Source: CAD feature listing. Evaluate the final solid. Frame: model axes, mm. A direction names the side the tool comes from. Give positions to 0.01 mm unless a question says otherwise; leave off trailing zeros. Loops run counter-clockwise (first coordinate to the right, second up) from the corner with the lowest first, then second, coordinate; pieces in that order, holes last. Notation, with made-up numbers: M 10,43.5 L 31,43.5 A30 ccw 31,77.5 Z; hole C 68,65 d9. An arc over 180 degrees is marked long. Answer in a Markdown table with one row per item.
```python
from build123d import *

# Parameters (mm, degrees)
SKETCH1_W           = 104
SKETCH1_H           = 6
BOSS_EXTRUDE1_DEPTH = 5
SKETCH2_W           = 104
SKETCH2_H           = 3
BOSS_EXTRUDE2_DEPTH = 92
SKETCH3_W           = 5
SKETCH3_H           = 6
BOSS_EXTRUDE3_DEPTH = 3
SKETCH4_W           = 5
SKETCH4_H           = 6
BOSS_EXTRUDE4_DEPTH = 3


with BuildPart() as part:
    # Sketch1 → Boss-Extrude1 (new body)
    with BuildSketch(Plane.XY):
        Rectangle(SKETCH1_W, SKETCH1_H)
    extrude(amount=-BOSS_EXTRUDE1_DEPTH)

    # Sketch2 → Boss-Extrude2 (add)
    with BuildSketch(Plane(origin=(0, 0, -5), x_dir=(-1, 0, 0), z_dir=(0, 0, -1))):
        with Locations((0, -1.5)):
            Rectangle(SKETCH2_W, SKETCH2_H)
    extrude(amount=BOSS_EXTRUDE2_DEPTH)

    # Sketch3 → Boss-Extrude3 (add)
    with BuildSketch(Plane(origin=(52, 0, 0), x_dir=(0, 0, -1), z_dir=(1, 0, 0))):
        with Locations((2.5, 0)):
            Rectangle(SKETCH3_W, SKETCH3_H)
    extrude(amount=BOSS_EXTRUDE3_DEPTH)

    # Sketch4 → Boss-Extrude4 (add)
    with BuildSketch(Plane.ZY.offset(52)):
        with Locations((-2.5, 0)):
            Rectangle(SKETCH4_W, SKETCH4_H)
    extrude(amount=BOSS_EXTRUDE4_DEPTH)


solid = part.part
```
1) Pin query (flat end, axial travel): pin 1 Ø3.5 at (y, z) = (-2, -58.5) entering from +X; pin 2 Ø4 at (x, z) = (40, -62.5) entering from +Y; pin 3 Ø2.5 at (y, z) = (-1.5, -69.5) entering from -X; pin 4 Ø2 at (x, y) = (20, 1.5) entering from +Z. Return the tip coordinate at first contact, or that it passes through.
Reply:
| item | result |
|---|---|
| pin 1 | stops at x = 52 |
| pin 2 | stops at y = 0 |
| pin 3 | stops at x = -52 |
| pin 4 | stops at z = 0 |
2) Section B-B, the plane x = 41. Return loops of the section in (y, z).
Reply:
| item | result |
|---|---|
| outline | M -3,-97 L 0,-97 L 0,-5 L 3,-5 L 3,0 L -3,0 Z |
3) Material intervals for L1, parallel to Y at x = -32, z = -50.5; L2, parallel to X at y = -0.9, z = -86; L3, parallel to Z at x = -48.5, y = 1.8, sorted ascending.
Reply:
| item | result |
|---|---|
| L1 | y = -3 to 0 |
| L2 | x = -52 to 52 |
| L3 | z = -5 to 0 |
4) Section A-A, the plane y = -1.5. Return loops of the section in (x, z), then the cut area to 3 significant figures.
Reply:
| item | result |
|---|---|
| outline | M -55,-5 L -52,-5 L -52,-97 L 52,-97 L 52,-5 L 55,-5 L 55,0 L -55,0 Z |
| area | 10,100 mm² |
5) Set-up query: faces 1 (the flat face through (1, 0, -50)), 2 (the flat face through (1, -3, -49)), 3 (the flat face through (-52, -2, -50)), 4 (the flat face through (52, -2, -50)), 5 (the flat face through (55, 0, -2)). Return all of +Z, -Z, +X, -X, +Y, -Y with unobstructed straight access to the full face (end or side cutting, diameter ignored); none if empty.
Reply:
| item | result |
|---|---|
| face 1 | -Z, +X, -X, +Y |
| face 2 | +Z, -Z, +X, -X, -Y |
| face 3 | -Z, -X, +Y, -Y |
| face 4 | -Z, +X, +Y, -Y |
| face 5 | +Z, -Z, +X, +Y, -Y |
6) Section C-C, the plane z = -60. Return loops of the section in (x, y), then the cut area to 3 significant figures.
Reply:
| item | result |
|---|---|
| outline | M -52,-3 L 52,-3 L 52,0 L -52,0 Z |
| area | 312 mm² |
